```python
from build123d import *

# Parameters (mm, degrees)
BOSS_EXTRUDE1_DEPTH                        = 2.54
SKETCH2_R                                  = 6.350000000000003
BOSS_EXTRUDE2_DEPTH                        = 25.4
MIRROR1_AT_THE_SECOND_PLANE_COPY_1_DEPTH   = 2.54
MIRROR1_AT_THE_SECOND_PLANE_COPY_2_SKETC_R = 6.350000000000003
MIRROR1_AT_THE_SECOND_PLANE_COPY_2_DEPTH   = 25.4
CHAMFER1_SIZE                              = 3.175
SKETCH3_R                                  = 1.5875000000000001
CUT_EXTRUDE1_DEPTH                         = 77.20000013333332
SKETCH4_R                                  = 2.0000000000000036
CUT_EXTRUDE2_DEPTH                         = 4.8
SKETCH5_R                                  = 1.5999999999999974
CUT_EXTRUDE3_DEPTH                         = 76.47674890287736
MIRROR2_AT_THE_SECOND_PLANE_COPY_1_SKETC_R = 2.0000000000000036
MIRROR2_AT_THE_SECOND_PLANE_COPY_1_DEPTH   = 4.8
MIRROR2_AT_THE_SECOND_PLANE_COPY_2_SKETC_R = 1.5999999999999974
MIRROR2_AT_THE_SECOND_PLANE_COPY_2_DEPTH   = 76.47674890287736
SKETCH6_R                                  = 3.1750000000000003
BOSS_EXTRUDE3_DEPTH                        = 3.175
MIRROR3_AT_THE_SECOND_PLANE_COPY_1_SKETC_R = 3.1750000000000003
MIRROR3_AT_THE_SECOND_PLANE_COPY_1_DEPTH   = 3.175


with BuildPart() as part:
    # Sketch1 → Boss-Extrude1 (new body)
    with BuildSketch(Plane(origin=(0, 0, 0), x_dir=(1, 0, 0), z_dir=(0, 1, 0))):
        with BuildLine():
            Line((-6.35, -7.8e-16), (0, 0))
            Line((0, 0), (0, 31.75))
            add(Edge.make_bspline(
                [(0, 31.75), (-11.810067101614626, 31.826488984199244), (-33.56352785361864, 50.29624659174145), (-44.09723296316762, 50.79019364197376)],
                knots=[0, 0, 0, 0, 0.9888261705717568, 0.9888261705717568, 0.9888261705717568, 0.9888261705717568], degree=3))
            ThreePointArc((-44.09723296316761, 50.79019364197375), (-39.836835647633734, 48.81362402803646), (-38.099999999999994, 44.44999999999999))
            ThreePointArc((-38.099999999999994, 44.44999999999999), (-39.959871939465415, 39.95987193946541), (-44.449999999999996, 38.09999999999999))
            add(Edge.make_bspline(
                [(-6.35, 19.05), (-6.175250797111612, 28.394037165914764), (-35.10270017916649, 38.03721238456326), (-44.449999999999996, 38.09999999999999)],
                knots=[0, 0, 0, 0, 1, 1, 1, 1], degree=3))
            Line((-6.35, 19.05), (-6.35, -7.8e-16))
        make_face()
        with BuildLine():
            add(Edge.make_bspline(
                [(-44.09723296316762, 50.79019364197376), (-44.216264829075314, 50.79577529044761), (-44.333864020357055, 50.79906156917483), (-44.45000000000001, 50.79999999999999)],
                knots=[0.9888261705717568, 0.9888261705717568, 0.9888261705717568, 0.9888261705717568, 1, 1, 1, 1], degree=3))
            ThreePointArc((-44.09723296316761, 50.79019364197375), (-44.27354834448691, 50.79754793705936), (-44.45000000000001, 50.79999999999999))
        make_face()
        with BuildLine():
            ThreePointArc((-38.099999999999994, 44.44999999999999), (-39.836835647633734, 48.81362402803646), (-44.09723296316761, 50.79019364197375))
            add(Edge.make_bspline(
                [(-44.09723296316762, 50.79019364197376), (-44.216264829075314, 50.79577529044761), (-44.333864020357055, 50.79906156917483), (-44.45000000000001, 50.79999999999999)],
                knots=[0.9888261705717568, 0.9888261705717568, 0.9888261705717568, 0.9888261705717568, 1, 1, 1, 1], degree=3))
            ThreePointArc((-44.45000000000001, 50.79999999999999), (-50.8, 44.44999999999998), (-44.449999999999996, 38.09999999999999))
            ThreePointArc((-44.449999999999996, 38.09999999999999), (-39.959871939465415, 39.95987193946541), (-38.099999999999994, 44.44999999999999))
        make_face()
    boss_extrude1 = extrude(amount=BOSS_EXTRUDE1_DEPTH)

    # Sketch2 → Boss-Extrude2 (add)
    with BuildSketch(Plane(origin=(0, 2.54, 0), x_dir=(1, 0, 0), z_dir=(0, 1, 0))):
        with Locations(Location((-44.449999999999996, 44.44999999999999, 0), (0, 0, 270))):
            Circle(SKETCH2_R)
    boss_extrude2 = extrude(amount=BOSS_EXTRUDE2_DEPTH)

    # Mirror1: Boss-Extrude1, Boss-Extrude2 across plane
    add(boss_extrude1.mirror(Plane(origin=(0, 0, 0), x_dir=(0, 0, 1), z_dir=(1, 0, 0))))
    add(boss_extrude2.mirror(Plane(origin=(0, 0, 0), x_dir=(0, 0, 1), z_dir=(1, 0, 0))))

    # Mirror1 at the second plane: Boss-Extrude1, Boss-Extrude2 across plane
    add(boss_extrude1.mirror(Plane.XY))
    add(boss_extrude2.mirror(Plane.XY))

    # Mirror1 at the second plane copy 1 sketc → Mirror1 at the second plane copy 1 (add)
    with BuildSketch(Plane(origin=(0, 0, 0), x_dir=(-1, 0, 0), z_dir=(0, 1, 0))):
        with BuildLine():
            Line((-6.35, -7.8e-16), (0, 0))
            Line((0, 0), (0, 31.75))
            add(Edge.make_bspline(
                [(0, 31.75), (-11.810067101614626, 31.826488984199244), (-33.56352785361864, 50.29624659174145), (-44.09723296316762, 50.79019364197376)],
                knots=[0, 0, 0, 0, 0.9888261705717568, 0.9888261705717568, 0.9888261705717568, 0.9888261705717568], degree=3))
            ThreePointArc((-44.09723296316761, 50.79019364197375), (-39.836835647633734, 48.81362402803646), (-38.099999999999994, 44.44999999999999))
            ThreePointArc((-38.099999999999994, 44.44999999999999), (-39.959871939465415, 39.95987193946541), (-44.449999999999996, 38.09999999999999))
            add(Edge.make_bspline(
                [(-6.35, 19.05), (-6.175250797111612, 28.394037165914764), (-35.10270017916649, 38.03721238456326), (-44.449999999999996, 38.09999999999999)],
                knots=[0, 0, 0, 0, 1, 1, 1, 1], degree=3))
            Line((-6.35, 19.05), (-6.35, -7.8e-16))
        make_face()
        with BuildLine():
            add(Edge.make_bspline(
                [(-44.09723296316762, 50.79019364197376), (-44.216264829075314, 50.79577529044761), (-44.333864020357055, 50.79906156917483), (-44.45000000000001, 50.79999999999999)],
                knots=[0.9888261705717568, 0.9888261705717568, 0.9888261705717568, 0.9888261705717568, 1, 1, 1, 1], degree=3))
            ThreePointArc((-44.09723296316761, 50.79019364197375), (-44.27354834448691, 50.79754793705936), (-44.45000000000001, 50.79999999999999))
        make_face()
        with BuildLine():
            ThreePointArc((-38.099999999999994, 44.44999999999999), (-39.836835647633734, 48.81362402803646), (-44.09723296316761, 50.79019364197375))
            add(Edge.make_bspline(
                [(-44.09723296316762, 50.79019364197376), (-44.216264829075314, 50.79577529044761), (-44.333864020357055, 50.79906156917483), (-44.45000000000001, 50.79999999999999)],
                knots=[0.9888261705717568, 0.9888261705717568, 0.9888261705717568, 0.9888261705717568, 1, 1, 1, 1], degree=3))
            ThreePointArc((-44.45000000000001, 50.79999999999999), (-50.8, 44.44999999999998), (-44.449999999999996, 38.09999999999999))
            ThreePointArc((-44.449999999999996, 38.09999999999999), (-39.959871939465415, 39.95987193946541), (-38.099999999999994, 44.44999999999999))
        make_face()
    extrude(amount=MIRROR1_AT_THE_SECOND_PLANE_COPY_1_DEPTH)

    # Mirror1 at the second plane copy 2 sketc → Mirror1 at the second plane copy 2 (add)
    with BuildSketch(Plane(origin=(0, 2.54, 0), x_dir=(-1, 0, 0), z_dir=(0, 1, 0))):
        with Locations(Location((-44.449999999999996, 44.44999999999999, 0), (0, 0, 270))):
            Circle(MIRROR1_AT_THE_SECOND_PLANE_COPY_2_SKETC_R)
    extrude(amount=MIRROR1_AT_THE_SECOND_PLANE_COPY_2_DEPTH)

    # Chamfer1
    chamfer1_edges = [part.edges().sort_by_distance(p)[0] for p in [
        (-44.449999999999996, 27.939999999999998, -50.79999999999999),
        (-44.449999999999996, 27.939999999999998, 50.79999999999999),
        (44.449999999999996, 27.939999999999998, -50.79999999999999),
        (44.449999999999996, 27.939999999999998, 50.79999999999999),
    ]]
    chamfer(chamfer1_edges, length=CHAMFER1_SIZE)

    # Sketch3 → Cut-Extrude1 (cut, through all)
    with BuildSketch(Plane(origin=(0, 2.54, 0), x_dir=(1, 0, 0), z_dir=(0, 1, 0))):
        with Locations(Location((0, 12.7, 0), (0, 0, 270))):
            Circle(SKETCH3_R)
        with Locations(Location((0, -12.7, 0), (0, 0, 270))):
            Circle(SKETCH3_R)
    extrude(amount=-CUT_EXTRUDE1_DEPTH, mode=Mode.SUBTRACT)

    # Sketch4 → Cut-Extrude2 (cut)
    with BuildSketch(Plane(origin=(0, 27.94, 0), x_dir=(1, 0, 0), z_dir=(0, 1, 0))):
        with Locations(Location((-44.449999999999996, 44.44999999999999, 0), (0, 0, 270))):
            Circle(SKETCH4_R)
    cut_extrude2 = extrude(amount=-CUT_EXTRUDE2_DEPTH, mode=Mode.SUBTRACT)

    # Sketch5 → Cut-Extrude3 (cut, through all)
    with BuildSketch(Plane(origin=(0, 23.14, 0), x_dir=(1, 0, 0), z_dir=(0, 1, 0))):
        with Locations(Location((-44.449999999999996, 44.44999999999999, 0), (0, 0, 270))):
            Circle(SKETCH5_R)
    cut_extrude3 = extrude(amount=-CUT_EXTRUDE3_DEPTH, mode=Mode.SUBTRACT)

    # Mirror2: Cut-Extrude2, Cut-Extrude3 across plane
    add(cut_extrude2.mirror(Plane(origin=(0, 0, 0), x_dir=(0, 0, 1), z_dir=(1, 0, 0))), mode=Mode.SUBTRACT)
    add(cut_extrude3.mirror(Plane(origin=(0, 0, 0), x_dir=(0, 0, 1), z_dir=(1, 0, 0))), mode=Mode.SUBTRACT)

    # Mirror2 at the second plane: Cut-Extrude2, Cut-Extrude3 across plane
    add(cut_extrude2.mirror(Plane.XY), mode=Mode.SUBTRACT)
    add(cut_extrude3.mirror(Plane.XY), mode=Mode.SUBTRACT)

    # Mirror2 at the second plane copy 1 sketc → Mirror2 at the second plane copy 1 (cut)
    with BuildSketch(Plane(origin=(0, 27.94, 0), x_dir=(-1, 0, 0), z_dir=(0, 1, 0))):
        with Locations(Location((-44.449999999999996, 44.44999999999999, 0), (0, 0, 270))):
            Circle(MIRROR2_AT_THE_SECOND_PLANE_COPY_1_SKETC_R)
    extrude(amount=-MIRROR2_AT_THE_SECOND_PLANE_COPY_1_DEPTH, mode=Mode.SUBTRACT)

    # Mirror2 at the second plane copy 2 sketc → Mirror2 at the second plane copy 2 (cut, through all)
    with BuildSketch(Plane(origin=(0, 23.14, 0), x_dir=(-1, 0, 0), z_dir=(0, 1, 0))):
        with Locations(Location((-44.449999999999996, 44.44999999999999, 0), (0, 0, 270))):
            Circle(MIRROR2_AT_THE_SECOND_PLANE_COPY_2_SKETC_R)
    extrude(amount=-MIRROR2_AT_THE_SECOND_PLANE_COPY_2_DEPTH, mode=Mode.SUBTRACT)

    # Sketch6 → Boss-Extrude3 (add)
    with BuildSketch(Plane(origin=(0, 2.54, 0), x_dir=(1, 0, 0), z_dir=(0, 1, 0))):
        with Locations(Location((-27.261721515519312, 38.55656577331098, 0), (0, 0, 270))):
            Circle(SKETCH6_R)
    boss_extrude3 = extrude(amount=BOSS_EXTRUDE3_DEPTH)

    # Mirror3: Boss-Extrude3 across plane
    add(boss_extrude3.mirror(Plane(origin=(0, 0, 0), x_dir=(0, 0, 1), z_dir=(1, 0, 0))))

    # Mirror3 at the second plane: Boss-Extrude3 across plane
    add(boss_extrude3.mirror(Plane.XY))

    # Mirror3 at the second plane copy 1 sketc → Mirror3 at the second plane copy 1 (add)
    with BuildSketch(Plane(origin=(0, 2.54, 0), x_dir=(-1, 0, 0), z_dir=(0, 1, 0))):
        with Locations(Location((-27.261721515519312, 38.55656577331098, 0), (0, 0, 270))):
            Circle(MIRROR3_AT_THE_SECOND_PLANE_COPY_1_SKETC_R)
    extrude(amount=MIRROR3_AT_THE_SECOND_PLANE_COPY_1_DEPTH)


solid = part.part
```
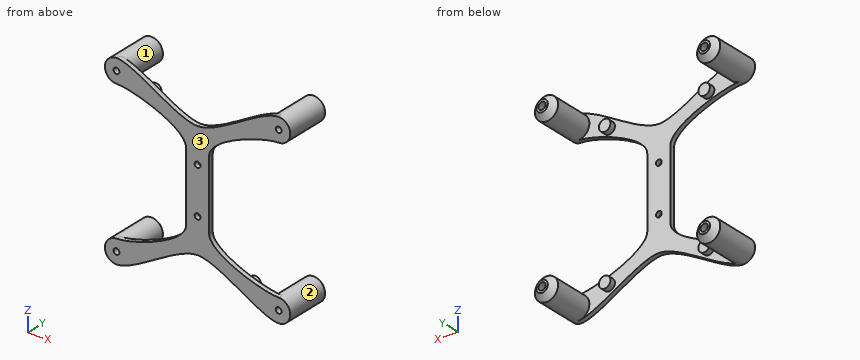
Work out the finished part from the listing and answer in its coordinate system (mm). Face numbers are marked on the shaded views. Round coordinates to 2 decimals unless told otherwise and drop trailing zeros. Write each loop counter-clockwise with the first axis right and the second up, starting at its lowest first coordinate (ties: lowest second). Pieces come first, ordered by that corner, then holes.
1) A cutting plane is placed at C-C on y = 4. Give the number of separate pieces and of enclosed holes in the cut face, and give its area (3 significant figures).
2) A cutting plane is placed at A-A on y = 19.5. Determine the outline of the cut face in (x, z), and give its area (3 significant figures).
3) Determine the mould class of the marked faces 1, 2 and 3 for opening direction Z: pulls with the +Z half, pulls with the -Z half, needs draft (parallel to the pull), parting line crosses it, or undercut.
4) Consider probe 1 along X at (y, z) = (24.35, 44.45); probe 2 along Z at (x, y) = (44.45, 16). Determine where each line is inside the solid, lowest interval first.
5) A cutting plane is placed at B-B on z = -12.7. Determine the outline of the cut face in (x, y).
6) Flat-ended cylindrical pins translate along their axes: P1, Ø7, axis at x = 26.5, z = 37.5, coming from the +Y side (3 decimals); P2, Ø1.3, axis at y = 1.5, z = -9.5, coming from the -X side; P3, Ø3.5, axis at x = 44.45, z = 44.45, coming from the +Y side. Find the tip coordinate at first contact, or state that the pin passes through.
7) A cutting plane is placed at D-D on z = 9.5. Determine the outline of the cut face in (x, y).
Entries:
1. separate pieces: 8
1. enclosed holes: 4
1. area: 601 mm2
2. outline: circle Ø12.7 at (-44.45, -44.45); circle Ø12.7 at (-44.45, 44.45); circle Ø12.7 at (44.45, -44.45); circle Ø12.7 at (44.45, 44.45); hole circle Ø3.2 at (-44.45, -44.45); hole circle Ø3.2 at (-44.45, 44.45); hole circle Ø3.2 at (44.45, -44.45); hole circle Ø3.2 at (44.45, 44.45)
2. area: 475 mm2
3. face 1: undercut
3. face 2: undercut
3. face 3: needs draft
4. probe 1: x = -50.8 to -46.45, -42.45 to -38.1, 38.1 to 42.45, 46.45 to 50.8
4. probe 2: z = -50.8 to -46.05, -42.85 to -38.1, 38.1 to 42.85, 46.05 to 50.8
5. outline: (-6.35, 0) - (-1.59, 0) - (-1.59, 2.54) - (-6.35, 2.54) - close; (1.59, 0) - (6.35, 0) - (6.35, 2.54) - (1.59, 2.54) - close
6. P1: stops at y = 5.715
6. P2: stops at x = -6.35
6. P3: stops at y = 23.14
7. outline: (-6.35, 0) - (6.35, 0) - (6.35, 2.54) - (-6.35, 2.54) - close
